CAD build for the part. Positions are in the model's coordinates, mm. Face numbers are marked on the shaded views. Give positions to 0.01 mm unless a question says otherwise; leave off trailing zeros. Write each loop counter-clockwise with the first axis right and the second up, starting at its lowest first coordinate (ties: lowest second). Pieces come first, ordered by that corner, then holes. Notation, with made-up numbers: (-25, -13.75) - (30, -13.75) arc R19 ccw to (30, 14.25) - close; hole circle Ø6 at (-13, 34.25). An arc over 180 degrees is marked (long way). Put each result on its own line as item: value. Start each with the question number.
1. Cut at B-B on z = 0. List the corners of the cut face in (x, y) (1 decimal), and give its area (3 significant figures).
2. Cut at A-A on x = 0. List the corners of the cut face in (y, z) (1 decimal), and give its area (3 significant figures).
3. Wall check: line 1 (Z direction, x = 0, y = -50.5) (1 decimal); line 2 (X direction, y = -32, z = -3); line 3 (Z direction, x = -2.5, y = -42.5). Give the ranges that are in metal, low to high.
4. Cut at C-C on y = -40.5. List the corners of the cut face in (x, z) (1 decimal).
5. Mould opens along Z. For the marked faces 1 and 2 say: +Z half, -Z half, draft (parallel to the pull), parting line (faces both ways), or undercut.
6. Drop a flat-ended pin along its axis: pin 1 (6 mm diameter, centred on x = 3.5, y = -48, fed in from +Z). Give the stop position or say it passes through.
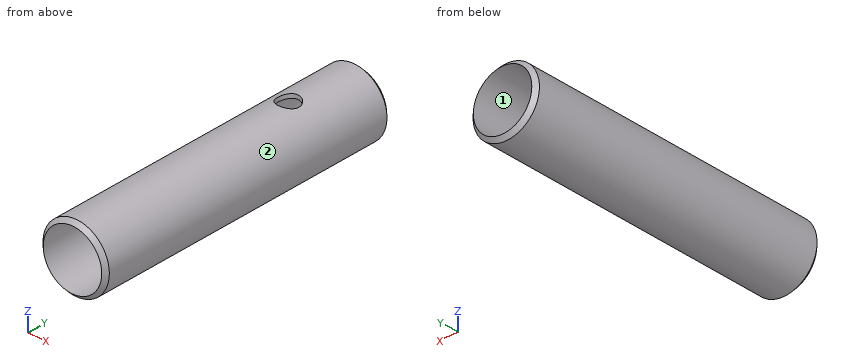
from build123d import *

# Parameters (mm, degrees)
F0_R     = 7.9375
F1_DEPTH = 76.2
F3_D     = 13.97
F3_DEPTH = 76.2
F3_TIP   = 4.1970114239
F7_D     = 5.08
F7_DEPTH = 25.4
F7_TIP   = 1.5261859723


# Not quite as in the source:
# - a fillet or chamfer that OpenCascade refuses, or shapes differently, is made with other operations: its cross-section is extruded or revolved along the edge and cut away or added


with BuildPart() as f1:
    # F0 (on Front) → F1 (new body)
    with BuildSketch(Plane.XZ):
        Circle(F0_R)
    extrude(amount=F1_DEPTH)

    # F3
    with Locations(Plane(origin=(0, 0, 0), x_dir=(1, 0, 0), z_dir=(0, 1, 0))):
        with Locations((0, 0)):
            Hole(F3_D / 2, depth=F3_DEPTH)
            with Locations((0, 0, -(F3_DEPTH + F3_TIP / 2))):  # 118° drill point
                Cone(0, F3_D / 2, F3_TIP, mode=Mode.SUBTRACT)

    # F4: chamfer of 1.778 on 1 edges, made by hand

    # F4_s1 → F4_t2 (revolve, cut)
    with BuildSketch(Plane.XY):
        Polygon((7.9375, -74.422), (6.1595, -76.2), (7.9375, -76.2), align=None)
    revolve(axis=Axis((0, -76.2, 0), (0, -1, 0)), mode=Mode.SUBTRACT)

    # F5: chamfer of 1.778 on 1 edges, made by hand

    # F5_s1 → F5_t2 (revolve, cut)
    with BuildSketch(Plane.XY):
        Polygon((7.9375, -1.778), (6.1595, 0), (7.9375, 0), align=None)
    revolve(axis=Axis((0, 0, 0), (0, -1, 0)), mode=Mode.SUBTRACT)

    # F7 (one way)
    with BuildSketch(Plane(origin=(0, 0, 0), x_dir=(1, 0, 0), z_dir=(0, 0, -1))):
        with Locations((0, 18.9180281013)):
            Circle(F7_D / 2)
    extrude(amount=-F7_DEPTH, mode=Mode.SUBTRACT)
    with Locations(Plane(origin=(0, 0, 0), x_dir=(1, 0, 0), z_dir=(0, 0, -1))):
        with Locations((0, 18.9180281013)):
            with Locations((0, 0, -(F7_DEPTH + F7_TIP / 2))):  # 118° drill point
                Cone(0, F7_D / 2, F7_TIP, mode=Mode.SUBTRACT)


solid = f1.part
Report:
1. outline: (-7.9, -74.4) - (-7, -75.4) - (-7, -0.8) - (-7.9, -1.8) - close; (7, -75.4) - (7.9, -74.4) - (7.9, -1.8) - (7, -0.8) - close
1. area: 140 mm²
2. outline: (-75.4, -7) - (-74.4, -7.9) - (-1.8, -7.9) - (-0.8, -7) - close; (-75.4, 7) - (-21.5, 7) - (-21.5, 7.9) - (-74.4, 7.9) - close; (-16.4, 7) - (-0.8, 7) - (-1.8, 7.9) - (-16.4, 7.9) - close
2. area: 135 mm²
3. line 1: z = -7.9 to -7, 7 to 7.9
3. line 2: x = -7.35 to -6.31, 6.31 to 7.35
3. line 3: z = -7.53 to -6.52, 6.52 to 7.53
4. outline: circle Ø15.9 at (0, 0); hole circle Ø14 at (0, 0)
5. face 1: undercut
5. face 2: parting line
6. pin 1: stops at z = 7.92
